```python
from build123d import *

# Parameters (mm, degrees)
BOSS_EXTRUDE1_DEPTH            = 6.35
M5_CLEARANCE_HOLE1_D           = 5.5
CBORE_FOR_M3_SHCS1_D           = 3.4
CBORE_FOR_M3_SHCS1_CBORE_D     = 6.5
CBORE_FOR_M3_SHCS1_CBORE_DEPTH = 3
CUT_EXTRUDE1_DEPTH             = 5.5


with BuildPart() as part:
    # Sketch1 → Boss-Extrude1 (new body)
    with BuildSketch(Plane.XY):
        with BuildLine():
            Line((5, 0), (20, 0))
            Line((20, 0), (20, -12.5))
            ThreePointArc((20, -12.5), (22.196699141, -17.803300859), (27.5, -20))
            Line((27.5, -20), (32.5, -20))
            ThreePointArc((32.5, -20), (37.803300859, -17.803300859), (40, -12.5))
            Line((40, -12.5), (40, 0))
            Line((40, 0), (55, 0))
            ThreePointArc((55, 0), (58.535533906, 1.464466094), (60, 5))
            Line((60, 5), (60, 35))
            ThreePointArc((60, 35), (58.535533906, 38.535533906), (55, 40))
            Line((55, 40), (5, 40))
            ThreePointArc((5, 40), (1.464466094, 38.535533906), (0, 35))
            Line((0, 35), (0, 5))
            ThreePointArc((0, 5), (1.464466094, 1.464466094), (5, 0))
        make_face()
    extrude(amount=BOSS_EXTRUDE1_DEPTH)

    # M5 Clearance Hole1 (through all)
    with Locations(Plane.XY.offset(6.35)):
        with Locations((30, -10), (10, 30), (50, 30)):
            Hole(M5_CLEARANCE_HOLE1_D / 2)

    # CBORE for M3 SHCS1 (through all)
    with Locations(Plane.XY.offset(6.35)):
        with Locations((38.396727498, 22.625800799), (54.396727498, 6.625800799), (38.396727498, 6.625800799), (54.396727498, 22.625800799), (22.396727498, 6.625800799), (22.396727498, 22.625800799)):
            CounterBoreHole(CBORE_FOR_M3_SHCS1_D / 2, CBORE_FOR_M3_SHCS1_CBORE_D / 2, CBORE_FOR_M3_SHCS1_CBORE_DEPTH)

    # Sketch7 → Cut-Extrude1 (cut)
    with BuildSketch(Plane(origin=(0, 0, 0), x_dir=(-1, 0, 0), z_dir=(0, 0, -1))):
        Polygon((-45.265727793, 30), (-47.632863896, 34.1), (-52.367136104, 34.1), (-54.734272207, 30), (-52.367136104, 25.9), (-47.632863896, 25.9), align=None)
        Polygon((-5.265727793, 30), (-7.632863896, 34.1), (-12.367136104, 34.1), (-14.734272207, 30), (-12.367136104, 25.9), (-7.632863896, 25.9), align=None)
        Polygon((-25.265727793, -10), (-27.632863896, -5.9), (-32.367136104, -5.9), (-34.734272207, -10), (-32.367136104, -14.1), (-27.632863896, -14.1), align=None)
    extrude(amount=-CUT_EXTRUDE1_DEPTH, mode=Mode.SUBTRACT)


solid = part.part
```
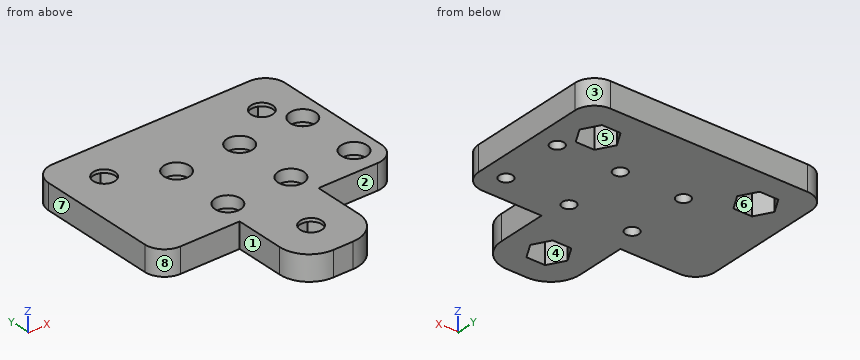
The listing builds one solid part. Answer for the finished solid, in the listing's coordinates (mm). Face numbers are marked on the shaded views. A direction names the side the tool comes from. Coordinates: 2 decimals unless noted, no trailing zeros. Loops run counter-clockwise (first coordinate to the right, second up) from the corner with the lowest first, then second, coordinate; pieces in that order, holes last. Notation, with made-up numbers: (29, 63.5) - (34, 63.5) arc R20 cw to (34, 96.5) - close; hole circle Ø2 at (62.25, 26.25). An arc over 180 degrees is marked (long way). Use a Markdown table: item, result. Add a question column.
1) The mould has two halves that part along Y. Classify the marked faces 5, 6, 7 and 8: released by +Y, released by -Y, zero draft, split by the parting line, or undercut.
2) Given pin 1 (2.5 mm diameter, centred on x = 22.4, y = 6.63, fed in from -Z); pin 2 (1.9 mm diameter, centred on x = 45.5, z = 2, fed in from -Y); pin 3 (5 mm diameter, centred on x = 55, y = 7, fed in from +Z); pin 4 (4 mm diameter, centred on x = 30, y = -12, fed in from -Z), each flat-ended and moving along its own axis, determine where each tip first touches the part or whether it passes through.
3) The part is cut by section B-B, the plane x = 50. Give the vertices of the cut face in (y, z), and give its area (3 significant figures).
4) For the marked faces 1, 2, 3 and 4, determine the directions among +Z, -Z, +X, -X, +Y, -Y from which every point of the face is accessible in a straight line to the end or side of a thin tool.
5) The part is cut by section C-C, the plane y = -1.5. Give the vertices of the cut face in (x, z), and give its area (3 significant figures).
6) The part is cut by section A-A, the plane x = 30. Give the vertices of the cut face in (y, z), and give its area (3 significant figures).
7) The part is cut by section D-D, the plane z = 4.5. State how many separate pieces and enclosed holes the cut face has, and give its area (3 significant figures).
8) Find the intervals of material crossed by line 1 (Y direction, x = 50, z = 5.8); line 2 (X direction, y = 21.5, z = 4.5); line 3 (X direction, y = 22, z = 5.75), in increasing order.
Here are the results:
| question | item | result |
|---|---|---|
| 1 | face 5 | undercut |
| 1 | face 6 | undercut |
| 1 | face 7 | zero draft |
| 1 | face 8 | released by -Y |
| 2 | pin 1 | passes through |
| 2 | pin 2 | stops at y = 0 |
| 2 | pin 3 | stops at z = 3.35 |
| 2 | pin 4 | stops at z = 5.5 |
| 3 | outline | (0, 0) - (25.9, 0) - (25.9, 5.5) - (27.25, 5.5) - (27.25, 6.35) - (0, 6.35) - close; (32.75, 5.5) - (34.1, 5.5) - (34.1, 0) - (40, 0) - (40, 6.35) - (32.75, 6.35) - close |
| 3 | area | 204 mm^2 |
| 4 | face 1 | +Z, -Z, -X, -Y |
| 4 | face 2 | +Z, -Z, +X, -Y |
| 4 | face 3 | +Z, -Z, +X, +Y |
| 4 | face 4 | -Z |
| 5 | outline | (20, 0) - (40, 0) - (40, 6.35) - (20, 6.35) - close |
| 5 | area | 127 mm^2 |
| 6 | outline | (-20, 0) - (-14.1, 0) - (-14.1, 5.5) - (-12.75, 5.5) - (-12.75, 6.35) - (-20, 6.35) - close; (-7.25, 5.5) - (-5.9, 5.5) - (-5.9, 0) - (40, 0) - (40, 6.35) - (-7.25, 6.35) - close |
| 6 | area | 331 mm^2 |
| 7 | separate pieces | 1 |
| 7 | enclosed holes | 9 |
| 7 | area | 2,380 mm^2 |
| 8 | line 1 | y = 0 to 27.25, 32.75 to 40 |
| 8 | line 2 | x = 0 to 19.35, 25.45 to 35.35, 41.45 to 51.35, 57.45 to 60 |
| 8 | line 3 | x = 0 to 19.21, 25.59 to 35.21, 41.59 to 51.21, 57.59 to 60 |
